from build123d import *

# Parameters (mm, degrees)
SKETCH1_R           = 9
BOSS_EXTRUDE1_DEPTH = 12.5
SKETCH2_R           = 2.5
CUT_EXTRUDE1_DEPTH  = 26
SKETCH3_R           = 4
CUT_EXTRUDE2_DEPTH  = 17.5


with BuildPart() as part:
    # Sketch1 → Boss-Extrude1 (new body, symmetric)
    with BuildSketch(Plane.XY):
        Circle(SKETCH1_R)
    extrude(amount=BOSS_EXTRUDE1_DEPTH, both=True)

    # Sketch2 → Cut-Extrude1 (cut, through all)
    with BuildSketch(Plane.XY.offset(12.5)):
        Circle(SKETCH2_R)
    extrude(amount=-CUT_EXTRUDE1_DEPTH, mode=Mode.SUBTRACT)

    # Sketch3 → Cut-Extrude2 (cut)
    with BuildSketch(Plane(origin=(0, 0, -12.5), x_dir=(-1, 0, 0), z_dir=(0, 0, -1))):
        Circle(SKETCH3_R)
    extrude(amount=-CUT_EXTRUDE2_DEPTH, mode=Mode.SUBTRACT)


solid = part.part
Source: CAD feature listing. Evaluate the final solid. Frame: model axes, mm. A direction names the side the tool comes from. Coordinates: 2 decimals unless noted, no trailing zeros. Loops run counter-clockwise (first coordinate to the right, second up) from the corner with the lowest first, then second, coordinate; pieces in that order, holes last. Notation, with made-up numbers: M 81.5,60 L 110.5,60 A22 ccw 110.5,96 Z; hole C -39,38.5 d7. An arc over 180 degrees is marked long. Answer in a Markdown table with one row per item.
Q1. Section C-C on z = 7.25. Return the cut outline in (x, y).
Answers below:
| item | result |
|---|---|
| outline | C 0,0 d18; hole C 0,0 d5 |
Q2. Set-up query: faces 1 (the cylindrical face through (0.867, -3.905, -3.873)), 2 (the flat face through (4, -2, -12.5)). Return all of +Z, -Z, +X, -X, +Y, -Y with unobstructed straight access to the full face (end or side cutting, diameter ignored); none if empty.
Answers below:
| item | result |
|---|---|
| face 1 | -Z |
| face 2 | -Z, +X, -X, +Y, -Y |
Q3. First-contact query: pin 1 (6.5 mm diameter, centred on x = 0, y = 0, fed in from +Z); pin 2 (4 mm diameter, centred on x = -1, y = -1.5, fed in from -Z); pin 3 (1 mm diameter, centred on x = 2, z = -0.5, fed in from +Y); pin 4 (4 mm diameter, centred on y = -2.5, z = 5.5, fed in from -X). Flat tips, straight axial feed; report the tip coordinate or a pass-through.
Answers below:
| item | result |
|---|---|
| pin 1 | stops at z = 12.5 |
| pin 2 | stops at z = 5 |
| pin 3 | stops at y = 8.87 |
| pin 4 | stops at x = -8.99 |
Q4. Ray query, probe 1 along Y at (x, z) = (0, 10.75); probe 2 along X at (y, z) = (-1, -7); probe 3 along Z at (x, y) = (3.75, 1). Return the intervals inside material, ascending. Write a range as from..to.
Answers below:
| item | result |
|---|---|
| probe 1 | y = -9..-2.5, 2.5..9 |
| probe 2 | x = -8.94..-3.87, 3.87..8.94 |
| probe 3 | z = 5..12.5 |
Q5. Draft query along X for faces 3 (the cylindrical face through (-1.172, 8.923, 0.175)), 4 (the flat face through (-2, 2, 5)), 5 (the flat face through (2, -2, 12.5)), 6 (the cylindrical face through (-0.54, -2.44, 8.8)). Return one class per face: pulls with the +X half, pulls with the -X half, needs draft (parallel to the pull), parting line crosses it, or undercut.
Answers below:
| item | result |
|---|---|
| face 3 | parting line crosses it |
| face 4 | undercut |
| face 5 | needs draft |
| face 6 | undercut |
Q6. Section D-D on y = 3.25. Return the cut outline in (x, z).
Answers below:
| item | result |
|---|---|
| outline | M -8.39,-12.5 L -2.33,-12.5 L -2.33,5 L 2.33,5 L 2.33,-12.5 L 8.39,-12.5 L 8.39,12.5 L -8.39,12.5 Z |
Q7. Section A-A on y = 0. Return the cut outline in (x, z), plus the area to 4 significant figures.
Answers below:
| item | result |
|---|---|
| outline | M -9,-12.5 L -4,-12.5 L -4,5 L -2.5,5 L -2.5,12.5 L -9,12.5 Z; M 2.5,5 L 4,5 L 4,-12.5 L 9,-12.5 L 9,12.5 L 2.5,12.5 Z |
| area | 272.5 mm^2 |
